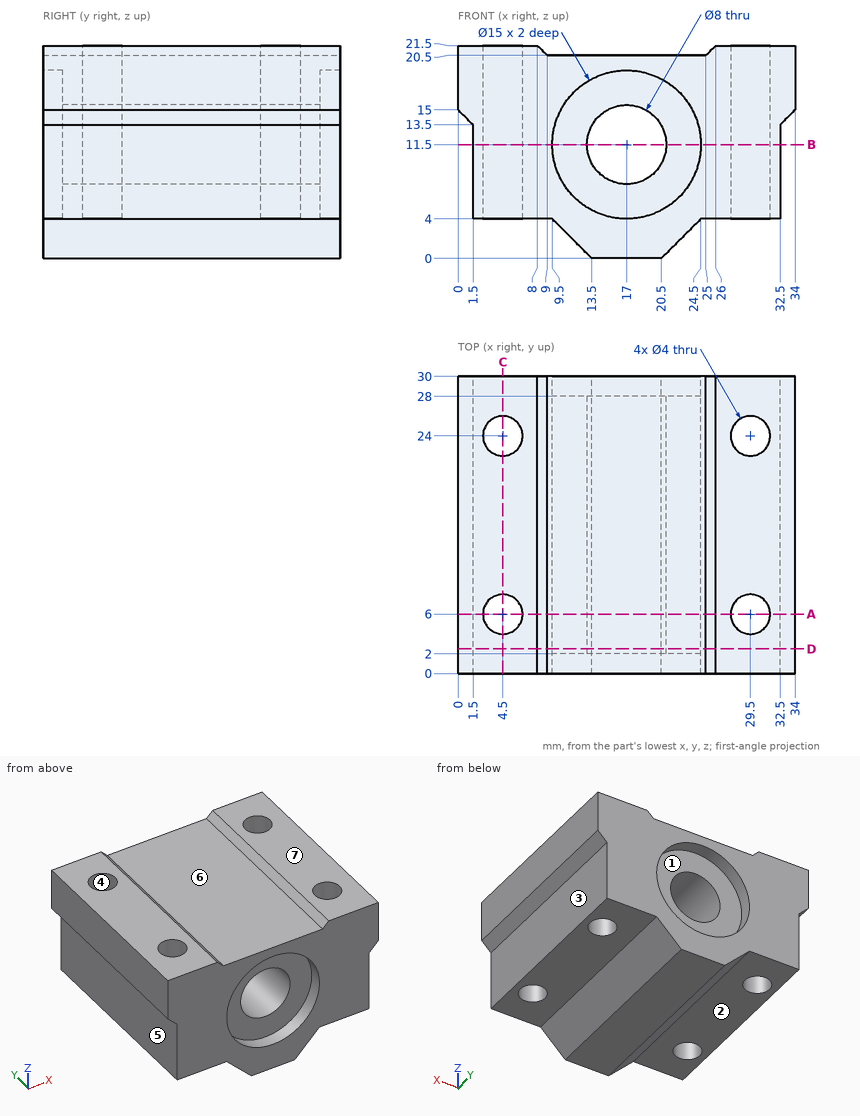
Answer from the drawing. Dimensions are ordinates in mm from the lowest x, y and z of the part. A direction names the side the tool comes from. Coordinates: 2 decimals unless noted, no trailing zeros. Order: outer loops, then holes, each group sorted by start corner. A loop starts at its lowest first (then second) coordinate and runs counter-clockwise, first axis right, second up. Notation, with made-up numbers: (38.5, 59) - (55.5, 59) arc R7 cw to (55.5, 64) - close; hole circle Ø5 at (73, 46). An arc over 180 degrees is marked (long way). Use one line per item in the form item = value.
(1) Which of the six approach directions +Z, -Z, +X, -X, +Y, -Y give full straight-line access (tool end or side, diameter ignored) to the marked faces 1, 2 and 3?
Computed values:
face_1 = +Y
face_2 = -Z, -X, +Y, -Y
face_3 = -Z, +X, +Y, -Y
(2) Given pin 1 Ø8 at (x, y) = (14.5, 16) entering from +Z; pin 2 Ø9 at (x, y) = (30, 13.5) entering from -Z; pin 3 Ø7.5 at (x, z) = (13.5, 12) entering from +Y, each flat-ended and moving along its own axis, determine where each tip first touches the part or whether it passes through.
Computed values:
pin_1 = 20.5
pin_2 = 4
pin_3 = 28
(3) Straight lines are drawn through the part: L1, parallel to Y at x = 4.5, z = 4.5; L2, parallel to X at y = 1.4, z = 11.5; L3, parallel to Y at x = 3.5, z = 20.5. For each, find the intervals that lie inside material, in ascending order.
Computed values:
L1 = 0 to 4, 8 to 22, 26 to 30
L2 = 1.5 to 9.5, 24.5 to 32.5
L3 = 0 to 4.27, 7.73 to 22.27, 25.73 to 30
(4) Section C-C, the plane x = 4.5 is taken. Give the vertices of the cut face in (y, z), then the cut area to 3 significant figures.
Computed values:
outline = (0, 4) - (4, 4) - (4, 21.5) - (0, 21.5) - close; (8, 4) - (22, 4) - (22, 21.5) - (8, 21.5) - close; (26, 4) - (30, 4) - (30, 21.5) - (26, 21.5) - close
area = 385 mm²
(5) For a pull along X with two mould halves and no side action, classify the marked faces 4, 5, 6 and 7 as pulls with the +X half, pulls with the -X half, needs draft (parallel to the pull), parting line crosses it, or undercut.
Computed values:
face_4 = undercut
face_5 = pulls with the -X half
face_6 = undercut
face_7 = needs draft
(6) Section D-D, the plane y = 2.5 is taken. Give the vertices of the cut face in (x, z).
Computed values:
outline = (0, 15) - (1.5, 13.5) - (1.5, 4) - (9.5, 4) - (13.5, 0) - (20.5, 0) - (24.5, 4) - (32.5, 4) - (32.5, 13.5) - (34, 15) - (34, 21.5) - (26, 21.5) - (25, 20.5) - (9, 20.5) - (8, 21.5) - (0, 21.5) - close; hole circle Ø8 at (17, 11.5)
(7) Section A-A, the plane y = 6 is taken. Give the vertices of the cut face in (x, z).
Computed values:
outline = (0, 15) - (1.5, 13.5) - (1.5, 4) - (2.5, 4) - (2.5, 21.5) - (0, 21.5) - close; (6.5, 4) - (9.5, 4) - (13.5, 0) - (20.5, 0) - (24.5, 4) - (27.5, 4) - (27.5, 21.5) - (26, 21.5) - (25, 20.5) - (9, 20.5) - (8, 21.5) - (6.5, 21.5) - close; (31.5, 4) - (32.5, 4) - (32.5, 13.5) - (34, 15) - (34, 21.5) - (31.5, 21.5) - close; hole circle Ø8 at (17, 11.5)
(8) Section B-B, the plane z = 11.5 is taken. Give the vertices of the cut face in (x, y).
Computed values:
outline = (1.5, 0) - (9.5, 0) - (9.5, 2) - (13, 2) - (13, 28) - (9.5, 28) - (9.5, 30) - (1.5, 30) - close; (21, 2) - (24.5, 2) - (24.5, 0) - (32.5, 0) - (32.5, 30) - (24.5, 30) - (24.5, 28) - (21, 28) - close; hole circle Ø4 at (4.5, 6); hole circle Ø4 at (4.5, 24); hole circle Ø4 at (29.5, 6); hole circle Ø4 at (29.5, 24)
